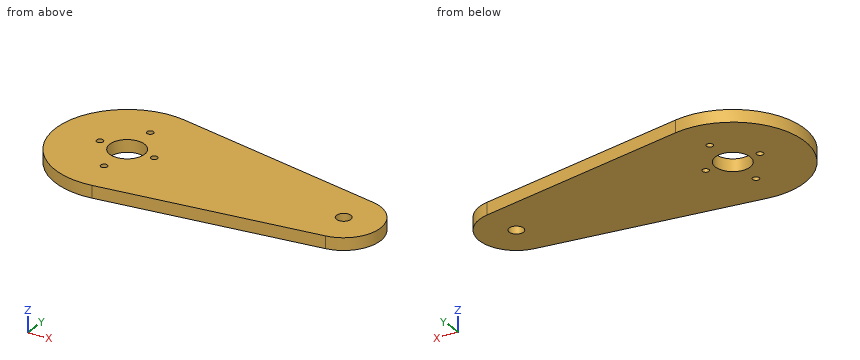
from build123d import *

# Parameters (mm, degrees)
SKETCH1_R           = 1.75
SKETCH1_R_2         = 4.25
SKETCH1_R_3         = 0.8
BOSS_EXTRUDE2_DEPTH = 3


with BuildPart() as part:
    # Sketch1 → Boss-Extrude2 (new body)
    with BuildSketch(Plane.XY):
        with BuildLine():
            Line((-17.329564893, 74.83964614), (35.264840048, 66.03177643))
            ThreePointArc((35.264840048, 66.03177643), (42.778052326, 57.084618151), (35.125066821, 48.256718465))
            Line((35.125066821, 48.256718465), (-17.601346169, 40.27703343))
            ThreePointArc((-17.601346169, 40.27703343), (-37.719458979, 57.717606069), (-17.329564893, 74.83964614))
        make_face()
        with Locations((33.778330565, 57.155386987)):
            Circle(SKETCH1_R, mode=Mode.SUBTRACT)
        with Locations((-20.22, 57.58)):
            Circle(SKETCH1_R_2, mode=Mode.SUBTRACT)
        with Locations((-13.47, 57.526921732)):
            Circle(SKETCH1_R_3, mode=Mode.SUBTRACT)
        with Locations((-26.97, 57.58)):
            Circle(SKETCH1_R_3, mode=Mode.SUBTRACT)
        with Locations((-20.22, 66.33)):
            Circle(SKETCH1_R_3, mode=Mode.SUBTRACT)
        with Locations((-20.22, 48.83)):
            Circle(SKETCH1_R_3, mode=Mode.SUBTRACT)
    extrude(amount=-BOSS_EXTRUDE2_DEPTH)


solid = part.part
CAD build for the part. Positions are in the model's coordinates, mm. Give positions to 0.01 mm unless a question says otherwise; leave off trailing zeros. Loops run counter-clockwise (first coordinate to the right, second up) from the corner with the lowest first, then second, coordinate; pieces in that order, holes last. Notation, with made-up numbers: M -33,10.25 L -8,10.25 A7 cw -8,14.25 Z; hole C -21.5,2 d4. An arc over 180 degrees is marked long. Answer in a Markdown table with one row per item. Add a question column.
Item 1: Drop flat-ended pins along their axis: P1, Ø1, axis at x = -20.22, y = 48.83, coming from the +Z side; P2, Ø1.5, axis at x = 24, z = -0.5, coming from the -Y side. Give the stop position or say it passes through.
Item 2: Band-saw the part on D-D on y = 71. Give the cut face in (x, z), then the cut area to 3 significant figures.
Item 3: Band-saw the part on B-B on z = -1.4. Give the cut face in (x, y).
Item 4: Probe probe 1 along Y at (x, z) = (-20.22, -1.15); probe 2 along X at (y, z) = (60, -2.15); probe 3 along Y at (x, z) = (-21.5, -1.85). List the from-to ranges inside material, lowest first.
Item 5: Band-saw the part on C-C on x = -3.5. Give the cut face in (y, z), then the cut area to 3 significant figures.
Item 6: Band-saw the part on A-A on x = -20.22. Give the cut face in (y, z), then the cut area to 3 significant figures.
Reply:
| question | item | result |
|---|---|---|
| 1 | P1 | passes through |
| 1 | P2 | stops at y = 46.46 |
| 2 | outline | M -31.45,-3 L 5.6,-3 L 5.6,0 L -31.45,0 Z |
| 2 | area | 111 mm^2 |
| 3 | outline | M -17.6,40.28 L 35.13,48.26 A9 ccw 35.26,66.03 L -17.33,74.84 A17.5 ccw long Z; hole C -26.97,57.58 d1.6; hole C -20.22,57.58 d8.5; hole C -20.22,48.83 d1.6; hole C -20.22,66.33 d1.6; hole C -13.47,57.53 d1.6; hole C 33.78,57.16 d3.5 |
| 4 | probe 1 | y = 40.08 to 48.03, 49.63 to 53.33, 61.83 to 65.53, 67.13 to 75.08 |
| 4 | probe 2 | x = -37.55 to -23.71, -16.73 to 42.32 |
| 4 | probe 3 | y = 40.13 to 53.53, 61.63 to 75.03 |
| 5 | outline | M 42.41,-3 L 72.52,-3 L 72.52,0 L 42.41,0 Z |
| 5 | area | 90.3 mm^2 |
| 6 | outline | M 40.08,-3 L 48.03,-3 L 48.03,0 L 40.08,0 Z; M 49.63,-3 L 53.33,-3 L 53.33,0 L 49.63,0 Z; M 61.83,-3 L 65.53,-3 L 65.53,0 L 61.83,0 Z; M 67.13,-3 L 75.08,-3 L 75.08,0 L 67.13,0 Z |
| 6 | area | 69.9 mm^2 |
